```python
from build123d import *

# Parameters (mm, degrees)
SKETCH_2_R          = 2.5
CUT_EXTRUDE_1_DEPTH = 10
SKETCH_3_R          = 2.5
CUT_EXTRUDE_2_DEPTH = 40.293765409


with BuildPart() as part:
    # 草图1 → 旋转1 (revolve)
    with BuildSketch(Plane.XY):
        Polygon((-10, 0), (14, 0), (14, -11), (2.2, -11), (2.2, -22), (0, -22), (0, -11), (-5, -11), (-5, -4.5), (-10, -4.5), align=None)
    revolve(axis=Axis((-10, 0, 0), (1, 0, 0)))

    # 草图2 → 切除-拉伸1 (cut)
    with BuildSketch(Plane.ZY):
        with Locations((0, 17.5)):
            Circle(SKETCH_2_R)
        with Locations((15.155444566, -8.75)):
            Circle(SKETCH_2_R)
        with Locations((-15.155444566, -8.75)):
            Circle(SKETCH_2_R)
    extrude(amount=-CUT_EXTRUDE_1_DEPTH, mode=Mode.SUBTRACT)

    # 草图3 → 切除-拉伸2 (cut, through all)
    with BuildSketch(Plane.ZY.offset(10)):
        Circle(SKETCH_3_R)
    extrude(amount=-CUT_EXTRUDE_2_DEPTH, mode=Mode.SUBTRACT)


solid = part.part
```
Model file for the job. Use its own axes, mm. A direction names the side the tool comes from. Coordinates: 2 decimals unless noted, no trailing zeros. Write each loop counter-clockwise with the first axis right and the second up, starting at its lowest first coordinate (ties: lowest second). Pieces come first, ordered by that corner, then holes. Notation, with made-up numbers: (12, 48.25) - (56, 48.25) arc R30 ccw to (56, 82.25) - close; hole circle Ø3 at (14.25, -18). An arc over 180 degrees is marked (long way). Use a Markdown table: item, result. Add a question column.
Item 1: Band-saw the part on A-A, the plane z = 0. Write the cut outline in (x, y).
Item 2: Band-saw the part on C-C, the plane z = -16. Write the cut outline in (x, y).
Item 3: Band-saw the part on D-D, the plane x = 7. Write the cut outline in (y, z), and give its area (3 significant figures).
Item 4: Two-plate mould, pull along Y, no slides. Class faces 1 (the face through (-7.54, 0.59, -4.46)), 2 (the face through (-10, -2, 2)), 3 (the face through (1.085, -9.708, -12.846)): pulls with the +Y half, pulls with the -Y half, needs draft (parallel to the pull), parting line crosses it, or undercut.
Item 5: Drill centre lines: line 1 along Y through (x, z) = (1.6, 0); line 2 along Z through (x, y) = (2, -8); line 3 along X through (y, z) = (-17, 2). Where is each one in solid material? Low to high.
Item 6: Drop flat-ended pins along their axis: pin 1 (3 mm diameter, centred on x = 0, z = 10, fed in from -Y); pin 2 (3 mm diameter, centred on y = 0, z = 0, fed in from -X); pin 3 (4 mm diameter, centred on y = 14, z = -2, fed in from +X); pin 4 (3 mm diameter, centred on y = 11.5, z = 17, fed in from -X). Give the stop position or say it passes through.
Item 7: 3-axis set-ups, long thin cutter, end or side, ignore diameter. For faces 4 (the face through (8.02, 2.38, 10.74)), 5 (the face through (1.08, -11.19, 14.61)), 6 (the face through (-5, 0, 5)): which of +Z, -Z, +X, -X, +Y, -Y reach the whole face in a straight line?
Item 8: Band-saw the part on B-B, the plane y = 0. Write the cut outline in (x, z), and give its area (3 significant figures).
A:
| question | item | result |
|---|---|---|
| 1 | outline | (-10, -4.5) - (-5, -4.5) - (-5, -11) - (0, -11) - (0, -22) - (2.2, -22) - (2.2, -11) - (14, -11) - (14, -2.5) - (-10, -2.5) - close; (-10, 2.5) - (14, 2.5) - (14, 11) - (2.2, 11) - (2.2, 15) - (0, 15) - (0, 11) - (-5, 11) - (-5, 4.5) - (-10, 4.5) - close; (0, 20) - (2.2, 20) - (2.2, 22) - (0, 22) - close |
| 2 | outline | (0, -15.1) - (2.2, -15.1) - (2.2, -11.1) - (0, -11.1) - close; (0, -6.4) - (2.2, -6.4) - (2.2, 15.1) - (0, 15.1) - close |
| 3 | outline | circle Ø22 at (0, 0); hole circle Ø5 at (0, 0) |
| 3 | area | 360 mm² |
| 4 | face 1 | parting line crosses it |
| 4 | face 2 | needs draft |
| 4 | face 3 | undercut |
| 5 | line 1 | y = -22 to -2.5, 2.5 to 15, 20 to 22 |
| 5 | line 2 | z = -20.49 to -17.54, -12.77 to 12.77, 17.54 to 20.49 |
| 5 | line 3 | x = 0 to 2.2 |
| 6 | pin 1 | stops at y = -20.29 |
| 6 | pin 2 | passes through |
| 6 | pin 3 | stops at x = 2.2 |
| 6 | pin 4 | stops at x = 0 |
| 7 | face 4 | +X |
| 7 | face 5 | +X, -X |
| 7 | face 6 | -X |
| 8 | outline | (-10, -4.5) - (-5, -4.5) - (-5, -11) - (0, -11) - (0, -22) - (2.2, -22) - (2.2, -11) - (14, -11) - (14, -2.5) - (-10, -2.5) - close; (-10, 2.5) - (14, 2.5) - (14, 11) - (2.2, 11) - (2.2, 22) - (0, 22) - (0, 11) - (-5, 11) - (-5, 4.5) - (-10, 4.5) - close |
| 8 | area | 391 mm² |
